from build123d import *

# Parameters (mm, degrees)
F1_DEPTH = 30
F3_DEPTH = 0.315
F4_SIZE2 = 0.173205
F4_SIZE  = 0.3


with BuildPart() as f1:
    # F0 (on Front) → F1 (new body)
    with BuildSketch(Plane.XZ):
        with BuildLine():
            ThreePointArc((0, 0.64), (0.187452, 0.187452), (0.64, 0))
            Line((0.64, 0), (11.36, 0))
            ThreePointArc((11.36, 0), (11.812548, 0.187452), (12, 0.64))
            Line((12, 0.64), (12, 3.86))
            ThreePointArc((12, 3.86), (11.812548, 4.312548), (11.36, 4.5))
            Line((11.36, 4.5), (0.64, 4.5))
            ThreePointArc((0.64, 4.5), (0.187452, 4.312548), (0, 3.86))
            Line((0, 3.86), (0, 0.64))
        make_face()
        with BuildLine():
            ThreePointArc((0.315, 3.86), (0.41019, 4.08981), (0.64, 4.185))
            Line((0.64, 4.185), (11.36, 4.185))
            ThreePointArc((11.36, 4.185), (11.58981, 4.08981), (11.685, 3.86))
            Line((11.685, 3.86), (11.685, 0.64))
            ThreePointArc((11.685, 0.64), (11.58981, 0.41019), (11.36, 0.315))
            Line((11.36, 0.315), (0.64, 0.315))
            ThreePointArc((0.64, 0.315), (0.41019, 0.41019), (0.315, 0.64))
            Line((0.315, 0.64), (0.315, 3.86))
        make_face(mode=Mode.SUBTRACT)
    extrude(amount=F1_DEPTH)

    # F2 (on face) → F3 (cut, through all)
    with BuildSketch(Plane(origin=(0, 0, 0), x_dir=(1, 0, 0), z_dir=(0, 0, -1))):
        with BuildLine():
            ThreePointArc((8.5, 13.4), (7.797056, 15.097056), (6.1, 15.8))
            Line((6.1, 15.8), (5.9, 15.8))
            ThreePointArc((5.9, 15.8), (4.202944, 15.097056), (3.5, 13.4))
            Line((3.5, 13.4), (3.5, 6.2))
            ThreePointArc((3.5, 6.2), (4.202944, 4.502944), (5.9, 3.8))
            Line((5.9, 3.8), (6.1, 3.8))
            ThreePointArc((6.1, 3.8), (7.797056, 4.502944), (8.5, 6.2))
            Line((8.5, 6.2), (8.5, 13.4))
        make_face()
    extrude(amount=-F3_DEPTH, mode=Mode.SUBTRACT)

    # F4
    f4_edges = [f1.edges().sort_by_distance(p)[0] for p in [
        (6, 0, 0),
        (6, -30, 0),
    ]]
    chamfer(f4_edges, length=F4_SIZE, length2=F4_SIZE2)


solid = f1.part
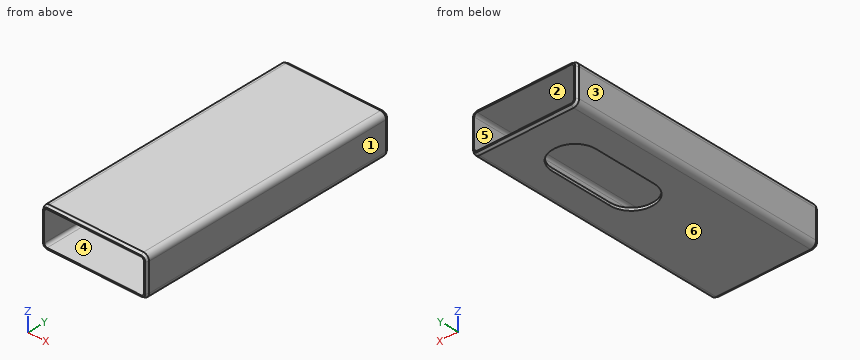
Geometry: final body of the model. Coordinates: model frame, mm. Face numbers are marked on the shaded views. A direction names the side the tool comes from. Give positions to 0.01 mm unless a question says otherwise; leave off trailing zeros. Write each loop counter-clockwise with the first axis right and the second up, starting at its lowest first coordinate (ties: lowest second). Pieces come first, ordered by that corner, then holes. Notation, with made-up numbers: (43.5, 67) - (76.5, 67) arc R18 cw to (76.5, 100) - close; hole circle Ø4 at (-10, -28.75). An arc over 180 degrees is marked (long way). Return JSON: item names as keys, results as strings. Group by question number.
1) Section C-C on z = 2.95. Return the cut outline in (x, y) (3 decimals).
2) Line query: line 1 (X direction, y = -21.5, z = 3.25) (3 decimals); line 2 (Z direction, x = 2.5, y = -23.5) (3 decimals); line 3 (Z direction, x = 7.75, y = -10) (3 decimals). Output: solid intervals per line, ascending.
3) Set-up query: the marked faces 1 and 2. Return all of +Z, -Z, +X, -X, +Y, -Y with unobstructed straight access to the full face (end or side cutting, diameter ignored); none if empty.
4) Mould query, pull axis X, two halves, no side actions, for the marked faces 3, 4, 5 and 6. Classes: released by +X, released by -X, zero draft, split by the parting line, or undercut.
5) Section B-B on y = -19. Return the cut outline in (x, z) (3 decimals).
6) Section D-D on y = -7. Return the cut outline in (x, z) (3 decimals), plus the area to 3 significant figures.
7) Section A-A on x = 3. Return the cut outline in (y, z) (3 decimals).
Filled in:
{
 "1": {"outline": "(0, -29.7) - (0.173, -30) - (0.315, -30) - (0.315, 0) - (0.173, 0) - (0, -0.3) - close; (11.685, -30) - (11.827, -30) - (12, -29.7) - (12, -0.3) - (11.827, 0) - (11.685, 0) - close"},
 "2": {"line 1": "x = 0 to 0.315, 11.685 to 12", "line 2": "z = 0 to 0.315, 4.185 to 4.5", "line 3": "z = 4.185 to 4.5"},
 "3": {"face 1": "+Z, -Z, +X, +Y, -Y", "face 2": "+Y, -Y"},
 "4": {"face 3": "released by -X", "face 4": "undercut", "face 5": "undercut", "face 6": "zero draft"},
 "5": {"outline": "(0, 0.64) arc R0.64 ccw to (0.64, 0) - (11.36, 0) arc R0.64 ccw to (12, 0.64) - (12, 3.86) arc R0.64 ccw to (11.36, 4.5) - (0.64, 4.5) arc R0.64 ccw to (0, 3.86) - close; hole (0.315, 0.64) arc R0.325 ccw to (0.64, 0.315) - (11.36, 0.315) arc R0.325 ccw to (11.685, 0.64) - (11.685, 3.86) arc R0.325 ccw to (11.36, 4.185) - (0.64, 4.185) arc R0.325 ccw to (0.315, 3.86) - close"},
 "6": {"outline": "(0, 0.64) arc R0.64 ccw to (0.64, 0) - (3.5, 0) - (3.5, 0.315) - (0.64, 0.315) arc R0.325 cw to (0.315, 0.64) - (0.315, 3.86) arc R0.325 cw to (0.64, 4.185) - (11.36, 4.185) arc R0.325 cw to (11.685, 3.86) - (11.685, 0.64) arc R0.325 cw to (11.36, 0.315) - (8.5, 0.315) - (8.5, 0) - (11.36, 0) arc R0.64 ccw to (12, 0.64) - (12, 3.86) arc R0.64 ccw to (11.36, 4.5) - (0.64, 4.5) arc R0.64 ccw to (0, 3.86) - close", "area": "8.16 mm^2"},
 "7": {"outline": "(-30, 0.173) - (-29.7, 0) - (-0.3, 0) - (0, 0.173) - (0, 0.315) - (-30, 0.315) - close; (-30, 4.185) - (0, 4.185) - (0, 4.327) - (-0.3, 4.5) - (-29.7, 4.5) - (-30, 4.327) - close"}
}
